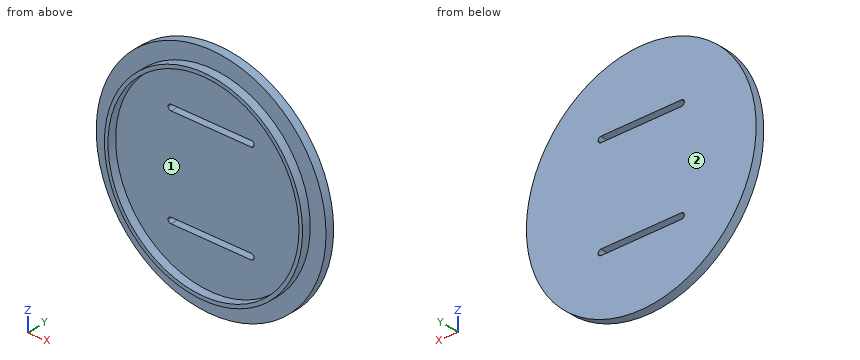
from build123d import *

# Parameters (mm, degrees)
F0_R     = 40
F1_DEPTH = 3
F2_R     = 34.5
F3_DEPTH = 3
F4_R     = 33.25
F5_DEPTH = 3
F7_DEPTH = 3.001


with BuildPart() as f1:
    # F0 (on Front) → F1 (new body)
    with BuildSketch(Plane.XZ):
        Circle(F0_R)
    extrude(amount=F1_DEPTH)

    # F2 (on face) → F3 (join)
    with BuildSketch(Plane.XZ.offset(3)):
        Circle(F2_R)
    extrude(amount=F3_DEPTH)

    # F4 (on face) → F5 (cut)
    with BuildSketch(Plane.XZ.offset(6)):
        Circle(F4_R)
    extrude(amount=-F5_DEPTH, mode=Mode.SUBTRACT)

    # F6 (on face) → F7 (cut, through all)
    with BuildSketch(Plane.XZ.offset(3)):
        with BuildLine():
            Line((14, 18.093938), (-14, 18.093938))
            ThreePointArc((-14, 18.093938), (-14.707107, 17.801045), (-15, 17.093938))
            ThreePointArc((-15, 17.093938), (-14.707107, 16.386831), (-14, 16.093938))
            Line((-14, 16.093938), (14, 16.093938))
            ThreePointArc((14, 16.093938), (14.707107, 16.386831), (15, 17.093938))
            ThreePointArc((15, 17.093938), (14.707107, 17.801045), (14, 18.093938))
        make_face()
        with BuildLine():
            Line((14, -16.093938), (-14, -16.093938))
            ThreePointArc((-14, -16.093938), (-14.707107, -16.386831), (-15, -17.093938))
            ThreePointArc((-15, -17.093938), (-14.707107, -17.801045), (-14, -18.093938))
            Line((-14, -18.093938), (14, -18.093938))
            ThreePointArc((14, -18.093938), (14.707107, -17.801045), (15, -17.093938))
            ThreePointArc((15, -17.093938), (14.707107, -16.386831), (14, -16.093938))
        make_face()
    extrude(amount=-F7_DEPTH, mode=Mode.SUBTRACT)


solid = f1.part
For this review, take the finished solid that the model builds, in its own axes (mm). Face numbers are marked on the shaded views. Round coordinates to 2 decimals unless told otherwise and drop trailing zeros. Order: outer loops, then holes, each group sorted by start corner. A loop starts at its lowest first (then second) coordinate and runs counter-clockwise, first axis right, second up. Notation, with made-up numbers: (65, -33) -> (113, -33) arc R22 cw to (113, -11) -> close; hole circle Ø11 at (60, 14.5). An arc over 180 degrees is marked (long way). Write item = value, one per line. Start each with the question number.
1) The part is to be moulded in two halves that separate along Z. For the marked faces 1 and 2, say which applies: +Z half, -Z half, draft (parallel to the pull), parting line (faces both ways), or undercut.
2) Take a section at A-A on x = 0. State the section outline as (y, z) points.
3) Take a section at B-B on y = -1.55. State the section outline as (x, z) points, plus the area to 3 significant figures.
4) Take a section at D-D on x = 24.5. State the section outline as (y, z) points.
5) To check wall thickness, follow line 1 (Z direction, x = 0, y = -5.2); line 2 (X direction, y = -3.35, z = 1); line 3 (Z direction, x = 13.5, y = -2.45). State the ranges of each line that lie inside material, in increasing order. Write a range as from..to.
6) Insertion check: pin 1 (1.5 mm diameter, centred on x = -22, y = -4.5, fed in from -Z); pin 2 (0.9 mm diameter, centred on x = -2, y = -2, fed in from -Z); pin 3 (8 mm diameter, centred on x = -16, z = -3, fed in from -Y). Each pin has a flat end and moves straight along its axis. Give the tip position at first contact, or say it passes through.
7) Take a section at C-C on z = 0. State the section outline as (x, y) points, plus the area to 4 significant figures.
Verdict:
q1.face_1 = undercut
q1.face_2 = draft
q2.outline = (-6, -34.5) -> (-3, -34.5) -> (-3, -40) -> (0, -40) -> (0, -18.09) -> (-3, -18.09) -> (-3, -33.25) -> (-6, -33.25) -> close; (-6, 33.25) -> (-3, 33.25) -> (-3, 18.09) -> (0, 18.09) -> (0, 40) -> (-3, 40) -> (-3, 34.5) -> (-6, 34.5) -> close; (-3, -16.09) -> (0, -16.09) -> (0, 16.09) -> (-3, 16.09) -> close
q3.outline = circle Ø80 at (0, 0); hole (-15, -17.09) arc R1 ccw to (-14, -18.09) -> (14, -18.09) arc R1 ccw to (15, -17.09) arc R1 ccw to (14, -16.09) -> (-14, -16.09) arc R1 ccw to start; hole (-15, 17.09) arc R1 ccw to (-14, 16.09) -> (14, 16.09) arc R1 ccw to (15, 17.09) arc R1 ccw to (14, 18.09) -> (-14, 18.09) arc R1 ccw to start
q3.area = 4,910 mm2
q4.outline = (-6, -24.29) -> (-3, -24.29) -> (-3, -31.62) -> (0, -31.62) -> (0, 31.62) -> (-3, 31.62) -> (-3, 24.29) -> (-6, 24.29) -> (-6, 22.48) -> (-3, 22.48) -> (-3, -22.48) -> (-6, -22.48) -> close
q5.line_1 = -34.5..-33.25, 33.25..34.5
q5.line_2 = -34.49..-33.23, 33.23..34.49
q5.line_3 = -37.65..-18.09, -16.09..16.09, 18.09..37.65
q6.pin_1 = -27.18
q6.pin_2 = -39.97
q6.pin_3 = -3
q7.outline = (-40, -3) -> (-34.5, -3) -> (-34.5, -6) -> (-33.25, -6) -> (-33.25, -3) -> (33.25, -3) -> (33.25, -6) -> (34.5, -6) -> (34.5, -3) -> (40, -3) -> (40, 0) -> (-40, 0) -> close
q7.area = 247.5 mm2
